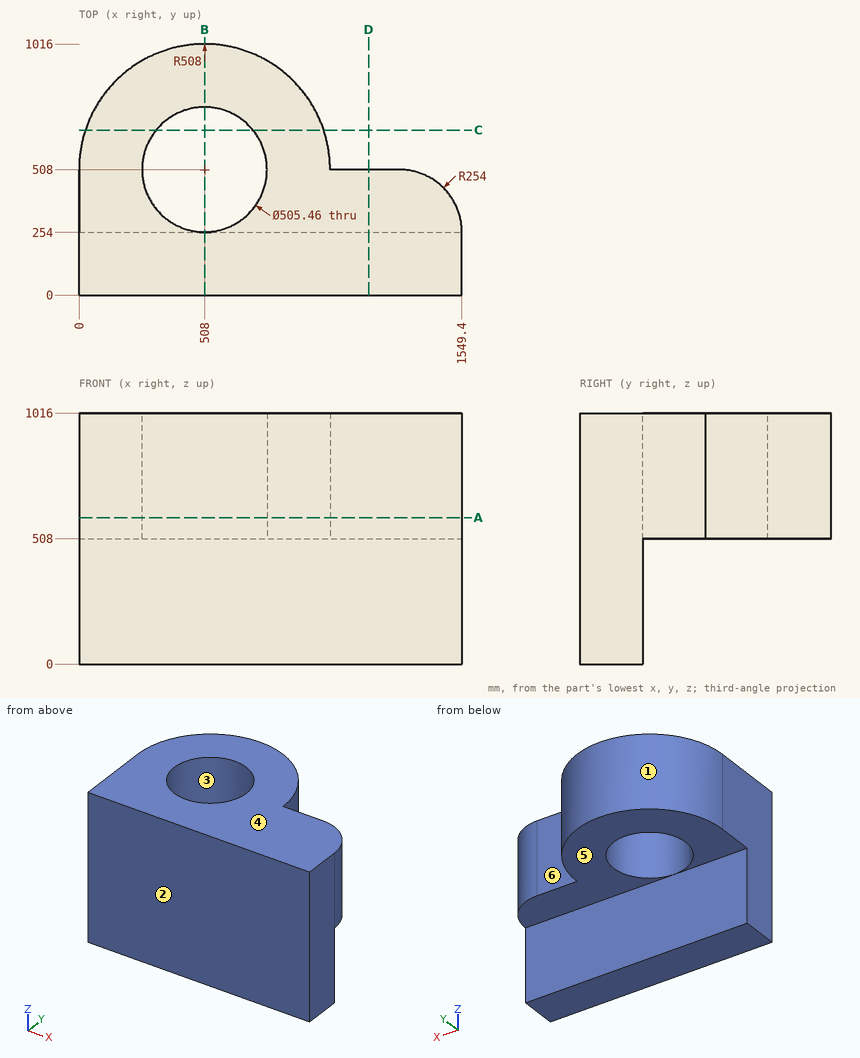
Here's the drawing with two shaded views (mm, measured from the low corner). I have some questions. A direction names the side the tool comes from. Coordinates: 2 decimals unless noted, no trailing zeros. Write each loop counter-clockwise with the first axis right and the second up, starting at its lowest first coordinate (ties: lowest second). Pieces come first, ordered by that corner, then holes. Notation, with made-up numbers: M 45.25,-9.75 L 88.25,-9.75 A31 cw 88.25,26.25 Z; hole C 57,-3.5 d4. An arc over 180 degrees is marked long. Answer as CSV lines item,"result".
Item 1: Please list where these lines run through material, in increasing order: line 1 along Y through (x, z) = (508, 656); line 2 along Y through (x, z) = (864, 484); line 3 along Z through (x, y) = (116.5, 632.5).
Geometry results:
line 1,"y = 0 to 255.27, 760.73 to 1016"
line 2,"y = 0 to 254"
line 3,"z = 508 to 1016"
Item 2: Imagine slicing it at A-A on z = 593.5. List the corners of the cut face in (x, y) for me, plus the area to 3 significant figures.
Geometry results:
outline,"M 0,0 L 1549.4,0 L 1549.4,254 A254 ccw 1295.4,508 L 1016,508 A508 ccw 0,508 Z; hole C 508,508 d505.46"
area,"978,000 mm2"
Item 3: I'm going to push flat-ended pins straight in: P1, Ø1.5, axis at x = 641.5, z = 598, coming from the +Y side; P2, Ø2, axis at y = 688.5, z = 670, coming from the -X side; P3, Ø5, axis at x = 818, z = 668.5, coming from the +Y side. Where does each tip first touch, or does it pass through?
Geometry results:
P1,"stops at y = 998.35"
P2,"stops at x = 32.77"
P3,"stops at y = 912.36"
Item 4: Imagine slicing it at D-D on x = 1172. List the corners of the cut face in (y, z) for me, plus the area to 3 significant figures.
Geometry results:
outline,"M 0,0 L 254,0 L 254,508 L 508,508 L 508,1016 L 0,1016 Z"
area,"387,000 mm2"
Item 5: On a 3-axis mill with a long thin cutter (end or side, diameter ignored), from which of +Z, -Z, +X, -X, +Y, -Y can I reach the whole of each face in a straight line? I mean the marked faces 4, 5 and 6. Say none if no direction works.
Geometry results:
face 4,"+Z, +X, -X, +Y, -Y"
face 5,"-Z, +X, -X, +Y"
face 6,"+Z, -Z, +X, +Y"
Item 6: Imagine slicing it at B-B on x = 508. List the corners of the cut face in (y, z) for me.
Geometry results:
outline,"M 0,0 L 254,0 L 254,508 L 255.27,508 L 255.27,1016 L 0,1016 Z; M 760.73,508 L 1016,508 L 1016,1016 L 760.73,1016 Z"
Item 7: We'd pull the mould along X, two halves only. Please class the marked faces 1, 2 and 3: +X half, -X half, draft (parallel to the pull), parting line (faces both ways), or undercut.
Geometry results:
face 1,"parting line"
face 2,"draft"
face 3,"undercut"
Item 8: Imagine slicing it at C-C on y = 667. List the corners of the cut face in (x, z) for me.
Geometry results:
outline,"M 25.52,508 L 311.55,508 L 311.55,1016 L 25.52,1016 Z; M 704.45,508 L 990.48,508 L 990.48,1016 L 704.45,1016 Z"
